from build123d import *

# Parameters (mm, degrees)
SKETCH5_R           = 22.225
SKETCH5_R_2         = 19.05
SKETCH6_R           = 22.225
SKETCH6_R_2         = 19.05
BOSS_EXTRUDE1_DEPTH = 76.2
SKETCH7_R           = 22.225
SKETCH7_R_2         = 19.05
BOSS_EXTRUDE2_DEPTH = 406.4


with BuildPart() as part:
    # Sweep1: sweep along a path in Sketch4
    with BuildLine(Plane.XY) as sweep1_path:
        ThreePointArc((56.324038217, 0), (39.827109367, 39.827109367), (0, 56.324038217))
    # Sketch5 → Sweep1 (sweep)
    with BuildSketch(Plane(origin=(0, 0, 0), x_dir=(1, 0, 0), z_dir=(0, 1, 0))):
        with Locations((56.324038217, 0)):
            Circle(SKETCH5_R)
        with Locations((56.324038217, 0)):
            Circle(SKETCH5_R_2, mode=Mode.SUBTRACT)
    sweep(path=sweep1_path.line)

    # Sketch6 → Boss-Extrude1 (add)
    with BuildSketch(Plane.ZY):
        with Locations((0, 56.324038217)):
            Circle(SKETCH6_R)
        with Locations((0, 56.324038217)):
            Circle(SKETCH6_R_2, mode=Mode.SUBTRACT)
    extrude(amount=BOSS_EXTRUDE1_DEPTH)

    # Sketch7 → Boss-Extrude2 (add)
    with BuildSketch(Plane.XZ):
        with Locations((56.324038217, 0)):
            Circle(SKETCH7_R)
        with Locations((56.324038217, 0)):
            Circle(SKETCH7_R_2, mode=Mode.SUBTRACT)
    extrude(amount=BOSS_EXTRUDE2_DEPTH)


solid = part.part
Verification items for the finished model (mm, model axes). A direction names the side the tool comes from. Give positions to 0.01 mm unless a question says otherwise; leave off trailing zeros. Loops run counter-clockwise (first coordinate to the right, second up) from the corner with the lowest first, then second, coordinate; pieces in that order, holes last. Notation, with made-up numbers: (17.5, 79) - (72.5, 79) arc R17 ccw to (72.5, 96) - close; hole circle Ø5 at (-30.75, 38.5). An arc over 180 degrees is marked (long way). Write item = value, one per line. Start each with the question number.
Q1. Thickness scan on line 1 (Z direction, x = 56.5, y = -373); line 2 (Y direction, x = -55.5, z = 0); line 3 (X direction, y = -318, z = -9). Record the ranges inside material, lowest first.
Q2. Tool access check on faces 1 (the face through (73, -406.4, 10)), 2 (the face through (34.12, -200.36, 0.98)), 3 (the face through (-37.57, 34.63, -4.82)). Record the directions out of +Z, -Z, +X, -X, +Y, -Y that give a thin tool (end or side, any length) a straight path to the whole face; none if there is none.
Q3. Cross-section at A-A, the plane z = 0. Enter the section's corners in (x, y), and give its area (3 significant figures).
Q4. Mould release check, pull along X, two halves, no side actions. Record for faces 4 (the face through (-76.2, 63.01, 18.01)), 5 (the face through (37.292, -200.355, 0.838)), 6 (the face through (-37.567, 37.727, -4.13)): released by +X, released by -X, zero draft, split by the parting line, or undercut.
Q5. Depth check by flat-ended pin: P1, Ø2, axis at y = -308.5, z = 3.5, coming from the +X side; P2, Ø4, axis at y = -59.5, z = 2.5, coming from the +X side; P3, Ø12, axis at x = 24, y = -1, coming from the -Z side; P4, Ø2, axis at x = 15, z = -17, coming from the -Y side. Enter the tip coordinate at first touch or a pass-through.
Q6. Cross-section at B-B, the plane y = -261. Enter the section's corners in (x, z) (3 decimals).
Answer key:
q1.line_1 = -22.22 to -19.05, 19.05 to 22.22
q1.line_2 = 34.1 to 37.27, 75.37 to 78.55
q1.line_3 = 36 to 39.53, 73.11 to 76.65
q2.face_1 = +Z, -Z, +X, -X, -Y
q2.face_2 = -Y
q2.face_3 = -X
q3.outline = (-76.2, 34.1) - (0, 34.1) arc R34.1 cw to (34.1, 0) - (34.1, -406.4) - (37.27, -406.4) - (37.27, 0) arc R37.27 ccw to (0, 37.27) - (-76.2, 37.27) - close; (-76.2, 75.37) - (0, 75.37) arc R75.37 cw to (75.37, 0) - (75.37, -406.4) - (78.55, -406.4) - (78.55, 0) arc R78.55 ccw to (0, 78.55) - (-76.2, 78.55) - close
q3.area = 3,630 mm^2
q4.face_4 = released by -X
q4.face_5 = undercut
q4.face_6 = zero draft
q5.P1 = 78.41
q5.P2 = 78.54
q5.P3 = through
q5.P4 = 37.98
q6.outline = circle Ø44.45 at (56.324, 0); hole circle Ø38.1 at (56.324, 0)
